```python
from build123d import *

# Parameters (mm, degrees)
SKETCH_1_R            = 50
EXTRUDE_1_DEPTH       = 7.7
SKETCH_2_R            = 2
CUT_EXTRUDE_1_DEPTH   = 7.7
SKETCH_3_R            = 14
SKETCH_3_R_2          = 10
EXTRUDE_1_2_DEPTH     = 100
SKETCH_4_R            = 74
SKETCH_4_R_2          = 30
CUT_EXTRUDE_1_2_DEPTH = 10


with BuildPart() as part:
    # 草图1 → Extrude 1 (new body)
    with BuildSketch(Plane.XY):
        with Locations(Location((0, 0, 0), (0, 0, 180))):
            Circle(SKETCH_1_R)
    extrude(amount=EXTRUDE_1_DEPTH)

    # 草图2 → Cut-Extrude 1 (cut)
    with BuildSketch(Plane.XY.offset(7.7)):
        with Locations((4.428990597, 16.671728833)):
            Circle(SKETCH_2_R)
        with Locations((16.652635993, 4.500246046)):
            Circle(SKETCH_2_R)
        with Locations((12.223645396, -12.171482787)):
            Circle(SKETCH_2_R)
        with Locations((-4.428990597, -16.671728833)):
            Circle(SKETCH_2_R)
        with Locations((-16.652635993, -4.500246046)):
            Circle(SKETCH_2_R)
        with Locations((-12.223645396, 12.171482787)):
            Circle(SKETCH_2_R)
    extrude(amount=-CUT_EXTRUDE_1_DEPTH, mode=Mode.SUBTRACT)

    # 草图3 → Extrude 1 2 (add)
    with BuildSketch(Plane.XY.offset(7.7)):
        Circle(SKETCH_3_R)
        Circle(SKETCH_3_R_2, mode=Mode.SUBTRACT)
    extrude(amount=EXTRUDE_1_2_DEPTH)

    # 草图4 → Cut-Extrude 1 2 (cut)
    with BuildSketch(Plane.XY.offset(7.7)):
        Circle(SKETCH_4_R)
        Circle(SKETCH_4_R_2, mode=Mode.SUBTRACT)
    extrude(amount=-CUT_EXTRUDE_1_2_DEPTH, mode=Mode.SUBTRACT)


solid = part.part
```
Geometry: final body of the model. Coordinates: model frame, mm. A direction names the side the tool comes from. Round coordinates to 2 decimals unless told otherwise and drop trailing zeros. Order: outer loops, then holes, each group sorted by start corner. A loop starts at its lowest first (then second) coordinate and runs counter-clockwise, first axis right, second up. Notation, with made-up numbers: (-13.5, -18) -> (32.5, -18) arc R15 ccw to (32.5, -10) -> close; hole circle Ø5 at (35, -14). An arc over 180 degrees is marked (long way). Use CSV: the item, a comma, the result in double quotes. Start each with the question number.
1) Section C-C (z = 55.5). Return the cut outline in (x, y), and give its area (3 significant figures).
2) First-contact query: pin 1 Ø5 at (x, y) = (-4.43, -16.67) entering from +Z; pin 2 Ø1.5 at (x, z) = (-2, 14.5) entering from +Y; pin 3 Ø1.5 at (x, z) = (4, 85) entering from +Y. Flat tips, straight axial feed; report the tip coordinate or a pass-through.
3) Section B-B (y = 0). Return the cut outline in (x, z).
4) Draft query along Y for faces 1 (the face through (0, 0, 0)), 2 (the face through (-4.69, -14.69, 3.9)), 3 (the face through (12.932, -5.362, 57)). Return one class per face: +Y half, -Y half, draft (parallel to the pull), parting line (faces both ways), or undercut.
5) Set-up query: faces 4 (the face through (18.56, 5.1, 3.9)), 5 (the face through (-6, 13, 7.7)). Return all of +Z, -Z, +X, -X, +Y, -Y with unobstructed straight access to the full face (end or side cutting, diameter ignored); none if empty.
6) Section A-A (x = -17.5). Return the cut outline in (y, z).
7) Material intervals for line 1 along Z through (x, y) = (-4, 26.5); line 2 along Y through (x, z) = (0, 87.5); line 3 along Y through (x, z) = (6, 8), sorted ascending. Write a range as from..to.
Returned:
1,outline,"circle Ø28 at (0, 0); hole circle Ø20 at (0, 0)"
1,area,"302 mm²"
2,pin 1,"stops at z = 7.7"
2,pin 2,"stops at y = 13.94"
2,pin 3,"stops at y = 13.62"
3,outline,"(-30, 0) -> (30, 0) -> (30, 7.7) -> (14, 7.7) -> (14, 107.7) -> (10, 107.7) -> (10, 7.7) -> (-10, 7.7) -> (-10, 107.7) -> (-14, 107.7) -> (-14, 7.7) -> (-30, 7.7) -> close"
4,face 1,"draft"
4,face 2,"undercut"
4,face 3,"parting line"
5,face 4,"+Z, -Z"
5,face 5,"+Z"
6,outline,"(-24.37, 0) -> (-6.31, 0) -> (-6.31, 7.7) -> (-24.37, 7.7) -> close; (-2.69, 0) -> (24.37, 0) -> (24.37, 7.7) -> (-2.69, 7.7) -> close"
7,line 1,"z = 0..7.7"
7,line 2,"y = -14..-10, 10..14"
7,line 3,"y = -12.65..-8, 8..12.65"
